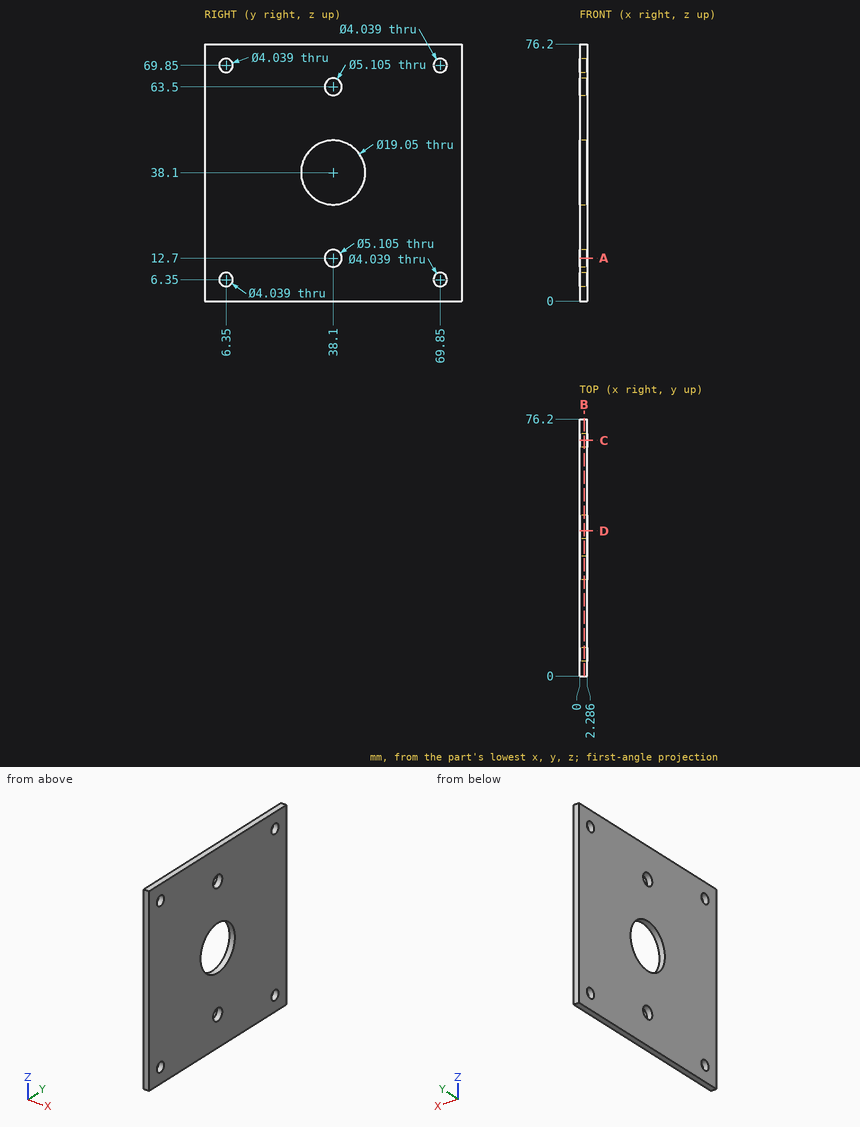
The figure shows three views and two pictorial views of one solid part (mm, origin at its lowest corner). Answer the questions. Coordinates: 2 decimals unless noted, no trailing zeros. Write each loop counter-clockwise with the first axis right and the second up, starting at its lowest first coordinate (ties: lowest second). Pieces come first, ordered by that corner, then holes.
1. The part is cut by section B-B, the plane x = 1.3. State how many separate pieces and enclosed holes the cut face has, and give its area (3 significant figures).
Results list:
separate pieces: 1
enclosed holes: 7
area: 5,430 mm2
2. Consider line 1 along Y through (x, z) = (1.6, 6.35); line 2 along Z through (x, y) = (2.1, 71.5) (1 decimal); line 3 along Z through (x, y) = (0.55, 39). Determine where each line is inside the solid, lowest interval first.
Results list:
line 1: y = 0 to 4.33, 8.37 to 67.83, 71.87 to 76.2
line 2: z = 0 to 5.2, 7.5 to 68.7, 71 to 76.2
line 3: z = 0 to 10.31, 15.09 to 28.62, 47.58 to 61.11, 65.89 to 76.2
3. A flat-ended cylindrical pin translates along its axis: pin 1 (4.5 mm diameter, centred on y = 38.1, z = 63.5, fed in from -X). Find the tip coordinate at first contact, or state that the pin passes through.
Results list:
pin 1: passes through
4. The part is cut by section D-D, the plane y = 43. Write down the section's boundary in (x, z), and give its area (3 significant figures).
Results list:
outline: (0, 0) - (2.29, 0) - (2.29, 29.93) - (0, 29.93) - close; (0, 46.27) - (2.29, 46.27) - (2.29, 76.2) - (0, 76.2) - close
area: 137 mm2
5. The part is cut by section C-C, the plane y = 69.85. Write down the section's boundary in (x, z), and give its area (3 significant figures).
Results list:
outline: (0, 0) - (2.29, 0) - (2.29, 4.33) - (0, 4.33) - close; (0, 8.37) - (2.29, 8.37) - (2.29, 67.83) - (0, 67.83) - close; (0, 71.87) - (2.29, 71.87) - (2.29, 76.2) - (0, 76.2) - close
area: 156 mm2
6. The part is cut by section A-A, the plane z = 12.7. Write down the section's boundary in (x, y).
Results list:
outline: (0, 0) - (2.29, 0) - (2.29, 35.55) - (0, 35.55) - close; (0, 40.65) - (2.29, 40.65) - (2.29, 76.2) - (0, 76.2) - close
